```python
from build123d import *

# Parameters (mm, degrees)
SKETCH_1_W                  = 86
SKETCH_1_H                  = 94.5
EXTRUDE_1_DEPTH             = 39.5
EXTRUDE_2_DEPTH             = 5
SKETCH_3_W                  = 80.6
SKETCH_3_H                  = 91.7
CUT_EXTRUDE_1_DEPTH         = 43.6
HOLE_WIZARD_8_3_8_3_1_D     = 8.3
HOLE_WIZARD_8_3_8_3_1_DEPTH = 3.2
FILLET_1_R                  = 3
SKETCH_7_R                  = 4.2
EXTRUDE_3_DEPTH             = 3.8
FILLET_2_R                  = 3
FILLET_3_R                  = 3
FILLET_4_R                  = 3
FILLET_5_R                  = 3
FILLET_6_R                  = 2


with BuildPart() as part:
    # Эскиз1 → Бобышка-Вытянуть1 (new body)
    with BuildSketch(Plane.XY.offset(22.25)):
        with Locations((47, 0)):
            Rectangle(SKETCH_1_W, SKETCH_1_H)
    extrude(amount=-EXTRUDE_1_DEPTH)

    # Эскиз2 → Бобышка-Вытянуть2 (add)
    with BuildSketch(Plane(origin=(0, 0, -17.25), x_dir=(-1, 0, 0), z_dir=(0, 0, -1))):
        with BuildLine():
            Line((-90, -47.25), (-90, -42.25))
            ThreePointArc((-90, -42.25), (-104, 0), (-90, 42.25))
            Line((-90, 42.25), (-90, 47.25))
            Line((-90, 47.25), (-4, 47.25))
            Line((-4, 47.25), (-4, -47.25))
            Line((-4, -47.25), (-90, -47.25))
        make_face()
        with BuildLine():
            Line((-90, -35.143201944), (-90, 35.143201944))
            ThreePointArc((-90, 35.143201944), (-100, 0), (-90, -35.143201944))
        make_face(mode=Mode.SUBTRACT)
    extrude(amount=EXTRUDE_2_DEPTH)

    # Эскиз3 → Вырез-Вытянуть1 (cut)
    with BuildSketch(Plane.XY.offset(22.25)):
        with Locations((48.3, 0)):
            Rectangle(SKETCH_3_W, SKETCH_3_H)
    extrude(amount=-CUT_EXTRUDE_1_DEPTH, mode=Mode.SUBTRACT)

    # Диаметр отверстия Ø8.3 (8.3)1
    with Locations(Plane.ZY.offset(-4)):
        with Locations((0, 0)):
            Hole(HOLE_WIZARD_8_3_8_3_1_D / 2, depth=HOLE_WIZARD_8_3_8_3_1_DEPTH)

    # Скругление1
    fillet_1_edges = [part.edges().sort_by_distance(p)[0] for p in [
        (4, -47.25, 0),
        (4, 47.25, 0),
    ]]
    fillet(fillet_1_edges, radius=FILLET_1_R)

    # Эскиз7 → Бобышка-Вытянуть3 (add)
    with BuildSketch(Plane.ZY.offset(-4)):
        Circle(SKETCH_7_R)
    extrude(amount=-EXTRUDE_3_DEPTH)

    # Скругление2
    fillet_2_edges = [part.edges().sort_by_distance(p)[0] for p in [
        (8, 0, -21.35),
    ]]
    fillet(fillet_2_edges, radius=FILLET_2_R)

    # Скругление3
    fillet_3_edges = [part.edges().sort_by_distance(p)[0] for p in [
        (8, -45.85, 1.95),
        (49.8, -45.85, -21.35),
        (8.878679656, -45.85, -20.471320344),
    ]]
    fillet(fillet_3_edges, radius=FILLET_3_R)

    # Скругление4
    fillet_4_edges = [part.edges().sort_by_distance(p)[0] for p in [
        (49.8, 45.85, -21.35),
        (8, 45.85, 1.95),
        (8.878679656, 45.85, -20.471320344),
    ]]
    fillet(fillet_4_edges, radius=FILLET_4_R)

    # Скругление5
    fillet_5_edges = [part.edges().sort_by_distance(p)[0] for p in [
        (88.6, -45.85, 1.95),
        (88.6, 0, -21.35),
        (88.6, -44.971320344, -20.471320344),
        (88.6, 45.85, 1.95),
        (88.6, 44.971320344, -20.471320344),
    ]]
    fillet(fillet_5_edges, radius=FILLET_5_R)

    # Скругление6
    fillet_6_edges = [part.edges().sort_by_distance(p)[0] for p in [
        (90, -38.696600972, -17.25),
        (90, 38.696600972, -17.25),
    ]]
    fillet(fillet_6_edges, radius=FILLET_6_R)


solid = part.part
```
Geometry: final body of the model. Coordinates: model frame, mm. A direction names the side the tool comes from. Coordinates: 2 decimals unless noted, no trailing zeros. Order: outer loops, then holes, each group sorted by start corner. A loop starts at its lowest first (then second) coordinate and runs counter-clockwise, first axis right, second up. Notation, with made-up numbers: (64, -31.75) -> (96, -31.75) arc R25 cw to (96, -8.75) -> close; hole circle Ø10 at (-31.5, -36). An arc over 180 degrees is marked (long way). Write each question's results on one line, items separated by ' | '. Start each with the question number.
1) Cut plane D-D, the plane y = -23. Output: boundary loops of the cut face in (x, z).
2) Cut plane C-C, the plane x = 29.5. Output: boundary loops of the cut face in (y, z), and give its area (3 significant figures).
3) Cut plane B-B, the plane y = -10.5. Output: boundary loops of the cut face in (x, z).
4) First-contact query: pin 1 (9.5 mm diameter, centred on x = 95.5, y = -5, fed in from +Z); pin 2 (20.5 mm diameter, centred on y = -10, z = 3, fed in from +X); pin 3 (5 mm diameter, centred on x = 31.5, y = -17.5, fed in from +Z). Flat tips, straight axial feed; report the tip coordinate or a pass-through.
5) Set-up query: faces 5 (the flat face through (100.2, -2.7, -17.25)), 6 (the flat face through (48, 45.85, 2)), 7 (the flat face through (48, 47.25, 0)). Return all of +Z, -Z, +X, -X, +Y, -Y with unobstructed straight access to the full face (end or side cutting, diameter ignored); none if empty.
6) Material intervals for line 1 along Y through (x, z) = (82, 2); line 2 along X through (y, z) = (-14.5, -16); line 3 along Z through (x, y) = (69, -28.5), sorted ascending.
7) Cut plane A-A, the plane z = 5.5. Output: boundary loops of the cut face in (x, y).
8) Mould query, pull axis X, two halves, no side actions, for faces 1 (the flat face through (48, -47.25, 0)), 2 (the cylindrical face through (103.997, -0.634, -19.479)), 3 (the flat face through (8, -1, 2)), 4 (the cylindrical face through (4.9, -46.39, -0.31)). Classes: released by +X, released by -X, zero draft, split by the parting line, or undercut.
Checks:
1) outline: (4, -22.25) -> (90, -22.25) -> (90, 22.25) -> (88.6, 22.25) -> (88.6, -18.35) arc R3 cw to (85.6, -21.35) -> (11, -21.35) arc R3 cw to (8, -18.35) -> (8, 22.25) -> (4, 22.25) -> close; (95.91, -22.25) -> (100.16, -22.25) -> (100.16, -17.25) -> (95.91, -17.25) -> close
2) outline: (-47.25, -22.25) -> (47.25, -22.25) -> (47.25, 22.25) -> (45.85, 22.25) -> (45.85, -18.35) arc R3 cw to (42.85, -21.35) -> (-42.85, -21.35) arc R3 cw to (-45.85, -18.35) -> (-45.85, 22.25) -> (-47.25, 22.25) -> close | area: 211 mm^2
3) outline: (4, -22.25) -> (90, -22.25) -> (90, 22.25) -> (88.6, 22.25) -> (88.6, -18.35) arc R3 cw to (85.6, -21.35) -> (11, -21.35) arc R3 cw to (8, -18.35) -> (8, 22.25) -> (4, 22.25) -> close; (99.17, -22.25) -> (103.22, -22.25) -> (103.22, -17.25) -> (99.17, -17.25) -> close
4) pin 1: z = -17.25 | pin 2: x = 90 | pin 3: z = -21.35
5) face 5: +Z, +X, +Y, -Y | face 6: +Z | face 7: +Z, -Z, +X, -X, +Y
6) line 1: -47.25 to -45.85, 45.85 to 47.25 | line 2: 4 to 8, 88.6 to 90 | line 3: -22.25 to -21.35
7) outline: (4, -44.25) arc R3 ccw to (7, -47.25) -> (90, -47.25) -> (90, 47.25) -> (7, 47.25) arc R3 ccw to (4, 44.25) -> close; hole (8, -42.85) arc R3 ccw to (11, -45.85) -> (85.6, -45.85) arc R3 ccw to (88.6, -42.85) -> (88.6, 42.85) arc R3 ccw to (85.6, 45.85) -> (11, 45.85) arc R3 ccw to (8, 42.85) -> close
8) face 1: zero draft | face 2: released by +X | face 3: undercut | face 4: released by -X
